Source: CAD feature listing. Evaluate the final solid. Frame: model axes, mm. Give positions to 0.01 mm unless a question says otherwise; leave off trailing zeros. Write each loop counter-clockwise with the first axis right and the second up, starting at its lowest first coordinate (ties: lowest second). Pieces come first, ordered by that corner, then holes. Notation, with made-up numbers: (35.25, 14) -> (48.25, 14) arc R8 cw to (48.25, 29) -> close; hole circle Ø5 at (-19.75, -30.5). An arc over 180 degrees is marked (long way). Use a Markdown table: item, result. Add a question column.
Autodesk Inventor part; units mm, degrees
ref_plane "YZ Plane" through (0, 0, 0) normal (1, 0, 0) x (0, 1, 0)
ref_plane "XZ Plane" through (0, 0, 0) normal (0, 1, 0) x (-1, 0, 0)
ref_plane "XY Plane" through (0, 0, 0) normal (0, 0, 1) x (1, 0, 0)
sketch "Эскиз1" plane through (0, 0, 0) normal (1, 0, 0) x (0, 1, 0)
  circle A0 centre (0, 0) radius 5
  dimension "d0" = 10
extrude "Выдавливание1" add sketch "Эскиз1" along normal blind 65
sketch "Эскиз2" plane through (0, 0, 0) normal (0, 0, 1) x (1, 0, 0)
  line L0 (0, 0) -> (12, 0)
  circle A0 centre (12, 0) radius 2
  line L1 (12, 0) -> (29, 0)
  line L2 (29, 0) -> (39, 0)
  circle A1 centre (39, 0) radius 1.5
  dimension "d3" = 12
  dimension "d4" = 4
  dimension "d5" = 17
  dimension "d6" = 10
  dimension "d7" = 3
extrude "Выдавливание2" cut sketch "Эскиз2" along normal mid plane 15.25
sketch "Эскиз3" plane through (0, 0, 0) normal (0, 1, 0) x (-1, 0, 0)
  line L0 (-40.5, -5) -> (-40.5, 5)
  line L1 (-37.5, -5) -> (-37.5, 5)
  line L2 (-37.5, 0) -> (-40.5, 0)
  circle A0 centre (-39, 0) radius 1.5
  point P0 (0, 0)
  dimension "d10" = 3
extrude "Выдавливание3" cut sketch "Эскиз3" along normal blind 15
thread "Резьба1"
thread "Резьба2"
sketch "Эскиз4" plane through (0, 0, 0) normal (0, 0, 1) x (1, 0, 0)
  line L0 (65, -5) -> (65, 5)
  line L1 (65, 0) -> (60, 0)
  circle A0 centre (60, 0) radius 1.5
  point P0 (0, 0)
  dimension "d17" = 5
  dimension "d18" = 3
extrude "Выдавливание4" cut sketch "Эскиз4" along normal mid plane 21.25
thread "Резьба3"
sketch "Эскиз5" plane through (0, 0, 0) normal (-1, 0, 0) x (0, 0, 1)
  point P0 (0, 0)
  point P1 (0, 0)
hole "Отверстие1" at (0, 0, 0) direction (1, 0, 0) diameter 2.459 depth 6 tip angle 118
properties part number "Вал ручки"
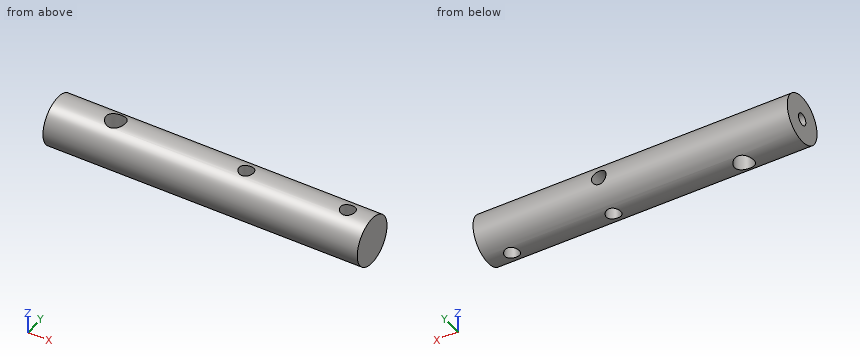
(1) First-contact query: pin 1 Ø1 at (y, z) = (-3, 0) entering from -X; pin 2 Ø1.8 at (x, y) = (39, 0) entering from -Z; pin 3 Ø1 at (x, z) = (14, -2.5) entering from +Y; pin 4 Ø3 at (x, y) = (23, 2) entering from -Z. Flat tips, straight axial feed; report the tip coordinate or a pass-through.
(2) Cut plane B-B on x = 39. Return the cut outline in (y, z).
(3) Cut plane D-D on x = 12. Return the cut outline in (y, z), then the cut area to 3 significant figures.
(4) Cut plane C-C on y = -4. Return the cut outline in (x, z).
(5) Cut plane A-A on z = 3. Return the cut outline in (x, y).
(6) Material intervals for L1, parallel to X at y = 0, z = -2.25; L2, parallel to X at y = 4.5, z = 0; L3, parallel to Z at x = 4.25, y = 0, sorted ascending.
Output:
| question | item | result |
|---|---|---|
| 1 | pin 1 | x = 0 |
| 1 | pin 2 | through |
| 1 | pin 3 | y = 4.58 |
| 1 | pin 4 | z = -4.97 |
| 2 | outline | (-1.5, -4.77) -> (-1.5, 4.77) arc R5 ccw to start; (1.5, -4.77) arc R5 ccw to (4.77, -1.5) -> (1.5, -1.5) -> close; (1.5, 1.5) -> (4.77, 1.5) arc R5 ccw to (1.5, 4.77) -> close |
| 3 | outline | (-2, -4.58) -> (-2, 4.58) arc R5 ccw to start; (2, -4.58) arc R5 ccw to (2, 4.58) -> close |
| 3 | area | 39.6 mm^2 |
| 4 | outline | (0, -3) -> (65, -3) -> (65, 3) -> (0, 3) -> close |
| 5 | outline | (0, -4) -> (65, -4) -> (65, 4) -> (0, 4) -> close; hole circle Ø4 at (12, 0); hole circle Ø3 at (39, 0); hole circle Ø3 at (60, 0) |
| 6 | L1 | 0 to 10, 14 to 37.5, 40.5 to 58.5, 61.5 to 65 |
| 6 | L2 | 0 to 37.5, 40.5 to 65 |
| 6 | L3 | -5 to -1.23, 1.23 to 5 |
